The model under review builds one solid part; all positions refer to its coordinate system, in mm. Face numbers are marked on the shaded views. A direction names the side the tool comes from. Coordinates: 2 decimals unless noted, no trailing zeros. Order: outer loops, then holes, each group sorted by start corner. A loop starts at its lowest first (then second) coordinate and runs counter-clockwise, first axis right, second up. Notation, with made-up numbers: (-28.75, 10.25) - (-11.75, 10.25) arc R24 cw to (-11.75, 43.25) - close; hole circle Ø3 at (68.25, -8.5). An arc over 180 degrees is marked (long way). Answer in a Markdown table with one row per item.
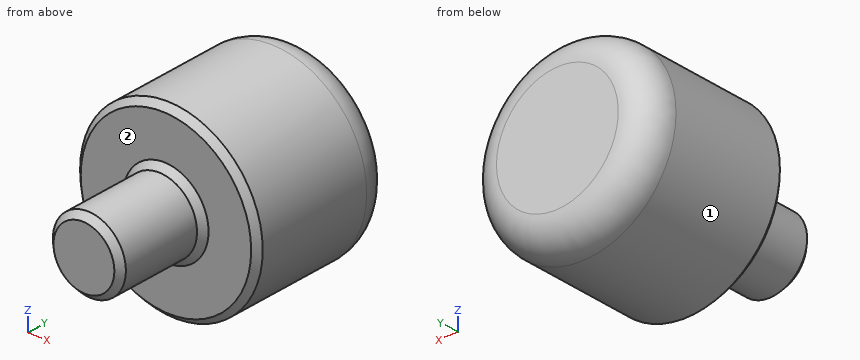
```python
from build123d import *

# Parameters (mm, degrees)
F0_R     = 15
F1_DEPTH = 25
F2_R     = 6
F3_DEPTH = 15
F4_R     = 5
F5_SIZE  = 1


with BuildPart() as f1:
    # F0 (on Front) → F1 (new body)
    with BuildSketch(Plane.XZ):
        Circle(F0_R)
    extrude(amount=F1_DEPTH)

    # F2 (on face) → F3 (join)
    with BuildSketch(Plane.XZ.offset(25)):
        Circle(F2_R)
    extrude(amount=F3_DEPTH)

    # F4
    f4_edges = [f1.edges().sort_by_distance(p)[0] for p in [
        (-15, 0, 0),
    ]]
    fillet(f4_edges, radius=F4_R)

    # F5
    f5_edges = [f1.edges().sort_by_distance(p)[0] for p in [
        (-6, -40, 0),
        (-6, -25, 0),
        (-15, -25, 0),
    ]]
    chamfer(f5_edges, length=F5_SIZE)


solid = f1.part
```
Item 1: We need section B-B, the plane x = 0. Write out the cut boundary in (y, z), then the cut area to 3 significant figures.
Check values:
| item | result |
|---|---|
| outline | (-40, -5) - (-39, -6) - (-26, -6) - (-25, -7) - (-25, -14) - (-24, -15) - (-5, -15) arc R5 ccw to (0, -10) - (0, 10) arc R5 ccw to (-5, 15) - (-24, 15) - (-25, 14) - (-25, 7) - (-26, 6) - (-39, 6) - (-40, 5) - close |
| area | 918 mm^2 |
Item 2: We need section A-A, the plane z = 0. Write out the cut boundary in (x, y).
Check values:
| item | result |
|---|---|
| outline | (-15, -24) - (-14, -25) - (-7, -25) - (-6, -26) - (-6, -39) - (-5, -40) - (5, -40) - (6, -39) - (6, -26) - (7, -25) - (14, -25) - (15, -24) - (15, -5) arc R5 ccw to (10, 0) - (-10, 0) arc R5 ccw to (-15, -5) - close |
Item 3: We need section D-D, the plane y = -29. Write out the cut boundary in (x, z), then the cut area to 3 significant figures.
Check values:
| item | result |
|---|---|
| outline | circle Ø12 at (0, 0) |
| area | 113 mm^2 |
Item 4: Clearance check with flat-ended pins moving along their axes: pin 1 Ø6 at (y, z) = (-29, -8) entering from +X; pin 2 Ø3 at (y, z) = (-33.5, -1.5) entering from -X; pin 3 Ø1 at (x, y) = (-8.5, -10.5) entering from -Z. State where each tip first meets the part, or that it passes through.
Check values:
| item | result |
|---|---|
| pin 1 | x = 3.32 |
| pin 2 | x = -6 |
| pin 3 | z = -12.69 |
Item 5: Tool access review of the marked faces 1 and 2: name each direction out of +Z, -Z, +X, -X, +Y, -Y from which nothing blocks a thin tool from reaching the whole face with its end or side.
Check values:
| item | result |
|---|---|
| face 1 | +Y, -Y |
| face 2 | -Y |
Item 6: We need section C-C, the plane y = -21. Write out the cut boundary in (x, z), then the cut area to 3 significant figures.
Check values:
| item | result |
|---|---|
| outline | circle Ø30 at (0, 0) |
| area | 707 mm^2 |
Item 7: To check wall thickness, follow line 1 (Y direction, x = -0.25, z = -9); line 2 (Z direction, x = 0.25, y = -20.5); line 3 (X direction, y = -14, z = -6). State the ranges of each line that lie inside material, in increasing order. Write a range as from..to.
Check values:
| item | result |
|---|---|
| line 1 | -25..0 |
| line 2 | -15..15 |
| line 3 | -13.75..13.75 |
